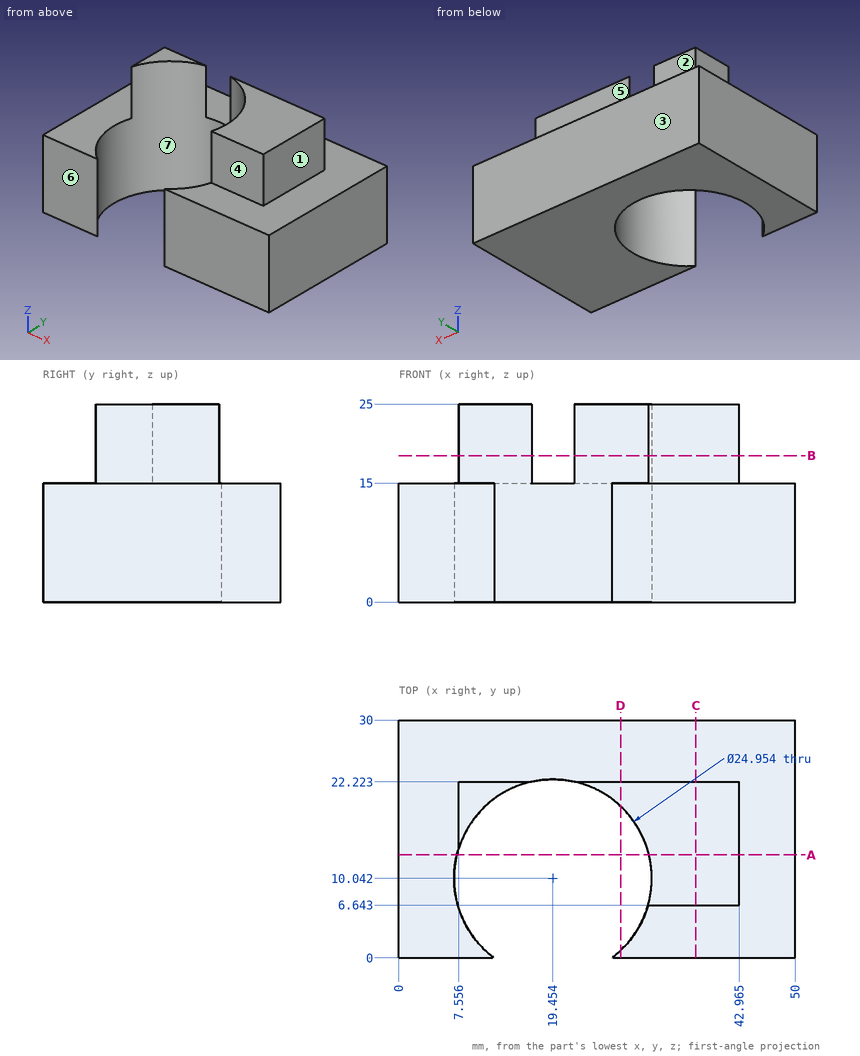
The drawing under review shows one solid part. Ordinate dimensions are in mm from its lowest x, y, z. A direction names the side the tool comes from. Give positions to 0.01 mm unless a question says otherwise; leave off trailing zeros. Order: outer loops, then holes, each group sorted by start corner. A loop starts at its lowest first (then second) coordinate and runs counter-clockwise, first axis right, second up. Notation, with made-up numbers: (5, 20) - (39, 20) arc R30 cw to (39, 51) - close; hole circle Ø9 at (56, 84). An arc over 180 degrees is marked (long way). Answer as a JSON object with one key per item and string values. Group by question number.
Item 1: Take a section at D-D on x = 28. Give the boundary of the cut face in (y, z), and give its area (3 significant figures).
Item 2: Take a section at C-C on x = 37.5. Give the boundary of the cut face in (y, z), and give its area (3 significant figures).
Item 3: Clearance check with flat-ended pins moving along their axes: pin 1 Ø1.5 at (x, y) = (42, 25) entering from +Z; pin 2 Ø5 at (y, z) = (14.5, 20) entering from +X (1 decimal); pin 3 Ø1.5 at (x, y) = (12, 19) entering from +Z; pin 4 Ø6.5 at (y, z) = (18, 22) entering from -X. State where each tip first meets the part, or that it passes through.
Item 4: Take a section at B-B on z = 18.5. Give the boundary of the cut face in (x, y) (1 decimal).
Item 5: Take a section at A-A on y = 13. Give the boundary of the cut face in (x, z) (1 decimal).
Item 6: Wall thickness on line 1 along Z through (x, y) = (47, 21); line 2 along X through (y, z) = (6, 7.25); line 3 along Y through (x, z) = (40.5, 17.5): over which ranges is each line inside the solid? List them lowest first.
Item 7: Machinability: for the marked faces 1, 2, 3 and 4, which of the approach directions +Z, -Z, +X, -X, +Y, -Y give a long, thin tool a straight path to every point of the face, cutting with its end or side? Answer none if there is none.
Item 8: Draft analysis for pull direction Y (two halves, no side actions). For the marked faces 5, 6 and 7, state which applies: pulls with the +Y half, pulls with the -Y half, needs draft (parallel to the pull), parting line crosses it, or undercut.
Reported:
{
 "1": {"outline": "(0, 0) - (0.95, 0) - (0.95, 15) - (0, 15) - close; (19.13, 0) - (30, 0) - (30, 15) - (22.22, 15) - (22.22, 25) - (19.13, 25) - close", "area": "208 mm^2"},
 "2": {"outline": "(0, 0) - (30, 0) - (30, 15) - (22.22, 15) - (22.22, 25) - (6.64, 25) - (6.64, 15) - (0, 15) - close", "area": "606 mm^2"},
 "3": {"pin 1": "z = 15", "pin 2": "x = 43", "pin 3": "through", "pin 4": "x = 7.56"},
 "4": {"outline": "(7.6, 13.8) arc R12.5 cw to (16.8, 22.2) - (7.6, 22.2) - close; (22.2, 22.2) arc R12.5 cw to (31.5, 6.6) - (43, 6.6) - (43, 22.2) - close"},
 "5": {"outline": "(0, 0) - (7.3, 0) - (7.3, 15) - (0, 15) - close; (31.6, 0) - (50, 0) - (50, 15) - (43, 15) - (43, 25) - (31.6, 25) - close"},
 "6": {"line 1": "0 to 15", "line 2": "0 to 7.65, 31.26 to 50", "line 3": "6.64 to 22.22"},
 "7": {"face 1": "+Z, +X, +Y, -Y", "face 2": "+Z, +X, -X, +Y", "face 3": "+Z, -Z, +X, -X, +Y", "face 4": "+Z, +X, -X, -Y"},
 "8": {"face 5": "pulls with the +Y half", "face 6": "pulls with the -Y half", "face 7": "undercut"}
}
